from build123d import *

# Parameters (mm, degrees)
EXTRUDE_START           = 21
EXTRUDE_1_DEPTH         = 42
CUT_EXTRUDE_4_OUTLINE_R = 2.1
CUT_EXTRUDE_4_DEPTH     = 20
EXTRUDE_2_DEPTH         = 2


# Read off the part's stored shape, not the designer's step: ｶｯﾄ - 押し出し4
with BuildPart() as part:
    # ｽｹｯﾁ2 → ﾎﾞｽ - 押し出し1 (new body)
    with BuildSketch(Plane.XY.offset(EXTRUDE_START)):
        with BuildLine():
            ThreePointArc((-75.5, 1), (-75.146446609, 1.146446609), (-75, 1.5))
            Line((-75, 1.5), (-75, 19))
            ThreePointArc((-75, 19), (-74.707106781, 19.707106781), (-74, 20))
            Line((-74, 20), (74, 20))
            ThreePointArc((74, 20), (74.707106781, 19.707106781), (75, 19))
            Line((75, 19), (75, 1.5))
            ThreePointArc((75, 1.5), (75.146446609, 1.146446609), (75.5, 1))
            Line((75.5, 1), (90.5, 1))
            ThreePointArc((90.5, 1), (90.853553391, 0.853553391), (91, 0.5))
            Line((91, 0.5), (91, 0))
            Line((91, 0), (-91, 0))
            Line((-91, 0), (-91, 0.5))
            ThreePointArc((-91, 0.5), (-90.853553391, 0.853553391), (-90.5, 1))
            Line((-90.5, 1), (-75.5, 1))
        make_face()
        with BuildLine():
            ThreePointArc((-27.5, 2), (-27.146446609, 2.146446609), (-27, 2.5))
            Line((-27, 2.5), (-27, 3.5))
            ThreePointArc((-27, 3.5), (-27.146446609, 3.853553391), (-27.5, 4))
            Line((-27.5, 4), (-46.5, 4))
            ThreePointArc((-46.5, 4), (-46.853553391, 3.853553391), (-47, 3.5))
            Line((-47, 3.5), (-47, 2.5))
            ThreePointArc((-47, 2.5), (-46.853553391, 2.146446609), (-46.5, 2))
            Line((-46.5, 2), (-27.5, 2))
        make_face(mode=Mode.SUBTRACT)
        with BuildLine():
            ThreePointArc((27, 2.5), (27.146446609, 2.146446609), (27.5, 2))
            Line((27.5, 2), (46.5, 2))
            ThreePointArc((46.5, 2), (46.853553391, 2.146446609), (47, 2.5))
            Line((47, 2.5), (47, 3.5))
            ThreePointArc((47, 3.5), (46.853553391, 3.853553391), (46.5, 4))
            Line((46.5, 4), (27.5, 4))
            ThreePointArc((27.5, 4), (27.146446609, 3.853553391), (27, 3.5))
            Line((27, 3.5), (27, 2.5))
        make_face(mode=Mode.SUBTRACT)
    extrude(amount=-EXTRUDE_1_DEPTH)

    # ｶｯﾄ - 押し出し4 outline → ｶｯﾄ - 押し出し4 (cut)
    with BuildSketch(Plane(origin=(0, 0, 0), x_dir=(1, 0, 0), z_dir=(0, 1, 0))):
        with BuildLine():
            ThreePointArc((-74, -21), (-74.214440627, -20.976737026), (-74.418904201, -20.908030435))
            Line((-74.418904201, -20.908030435), (-91, -14))
            Line((-91, -14), (-91, -21))
            Line((-91, -21), (-74, -21))
        make_face()
        with BuildLine():
            ThreePointArc((74.488899944, -20.872339868), (74.252646128, -20.96755875), (74, -21))
            Line((74, -21), (91, -21))
            Line((91, -21), (91, -14))
            Line((91, -14), (74.488899944, -20.872339868))
        make_face()
        Polygon((-74.21393, 21), (-91, 21), (-91, 14), align=None)
        with BuildLine():
            Line((-91, 2.1), (-91, -2.1))
            Line((-91, -2.1), (-82.5, -2.1))
            ThreePointArc((-82.5, -2.1), (-80.4, 0), (-82.5, 2.1))
            Line((-82.5, 2.1), (-91, 2.1))
        make_face()
        with BuildLine():
            Line((91, 21), (74, 21))
            ThreePointArc((74, 21), (74.260916595, 20.965361347), (74.503757591, 20.863845061))
            Line((74.503757591, 20.863845061), (91, 14))
            Line((91, 14), (91, 21))
        make_face()
        with Locations((82.5, 0)):
            Circle(CUT_EXTRUDE_4_OUTLINE_R)
    extrude(amount=CUT_EXTRUDE_4_DEPTH, mode=Mode.SUBTRACT)

    # ｽｹｯﾁ5 → ﾎﾞｽ - 押し出し2 (add)
    with BuildSketch(Plane(origin=(75, 0, 0), x_dir=(0, 0, -1), z_dir=(1, 0, 0))):
        with BuildLine():
            Line((-8.925734, 3), (8.925734, 3))
            ThreePointArc((8.925734, 3), (10.240738094, 3.303564532), (11.289616453, 4.152823844))
            ThreePointArc((11.289616453, 4.152823844), (12.612818852, 8.006934379), (11.275142981, 11.856045429))
            ThreePointArc((11.275142981, 11.856045429), (10.228153822, 12.698901284), (8.918218, 13))
            Line((8.918218, 13), (-8.918218, 13))
            ThreePointArc((-8.918218, 13), (-10.228153822, 12.698901284), (-11.275142981, 11.856045429))
            ThreePointArc((-11.275142981, 11.856045429), (-12.612818852, 8.006934379), (-11.289616453, 4.152823844))
            ThreePointArc((-11.289616453, 4.152823844), (-10.240738094, 3.303564532), (-8.925734, 3))
        make_face()
    extrude(amount=EXTRUDE_2_DEPTH)


solid = part.part
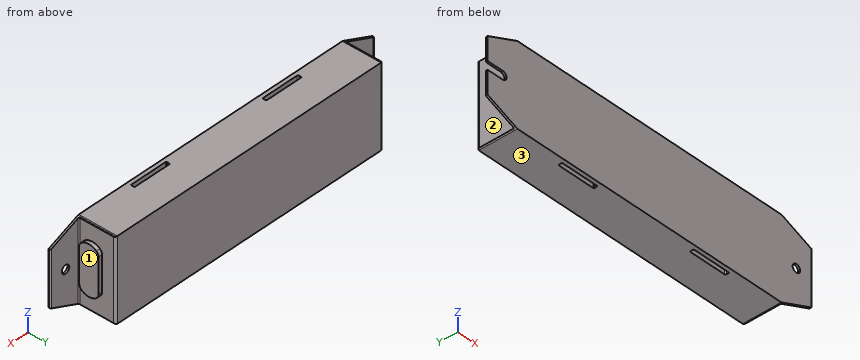
For this review, take the finished solid that the model builds, in its own axes (mm). Face numbers are marked on the shaded views. A direction names the side the tool comes from. Coordinates: 2 decimals unless noted, no trailing zeros. Order: outer loops, then holes, each group sorted by start corner. A loop starts at its lowest first (then second) coordinate and runs counter-clockwise, first axis right, second up. Notation, with made-up numbers: (83, 44) - (137, 44) arc R21 ccw to (137, 74) - close; hole circle Ø2 at (19.25, 37.5). An arc over 180 degrees is marked (long way). Use one line per item in the form item = value.
Q1. For the marked faces 1, 2 and 3, list the 3-axis set-ups (+Z, -Z, +X, -X, +Y, -Y) from which the entire face can be reached by the end or side of a thin tool; tool diameter is ignored.
Checked values:
face_1 = +Z, -Z, +X, +Y
face_2 = +Z, -Z, -X, +Y
face_3 = -Z, +X, -X, +Y, -Y
Q2. For probe 1 along X at (y, z) = (3.5, 4.5); probe 2 along Y at (x, z) = (-38.5, -9.5); probe 3 along X at (y, z) = (0.4, 0), list the stretches that pass through material, from the lowest coordinate up. Write a range as from..to.
Checked values:
probe_1 = -75..-47, -27..27, 47..77
probe_2 = 0..2, 4..20
probe_3 = -80.4..80.4, 84.6..91
Q3. Consider section A-A (z = -7). Give the number of separate pieces and of enclosed holes in the cut face, then the cut area to 3 significant figures.
Checked values:
separate_pieces = 1
enclosed_holes = 2
area = 2,970 mm2
Q4. For P1, Ø6, axis at y = 9, z = -16, coming from the -X side; P2, Ø12, axis at x = -83, z = -4.5, coming from the +Y side; P3, Ø2, axis at x = 58.5, z = -10.5, coming from the -Y side; P4, Ø11, axis at y = 8.5, z = 0.5, coming from the +X side, all flat-tipped, find the tip position at first contact; note any pin that passes through.
Checked values:
P1 = -75
P2 = 1
P3 = 0
P4 = 77
Q5. Consider section C-C (x = 82.5). Give the boundary of the cut face in (y, z).
Checked values:
outline = (0, -17.54) - (1, -17.54) - (1, -2.1) - (0, -2.1) - close; (0, 2.1) - (1, 2.1) - (1, 17.54) - (0, 17.54) - close
